from build123d import *

# Parameters (mm, degrees)
F4_R      = 12.7
F5_DEPTH  = 25.4
F7_R      = 12.7
F8_DEPTH  = 25.4
F9_R      = 7.463803
F9_R_2    = 6.828803
F10_DEPTH = 0.635


with BuildPart() as f1:
    # F0 (on Front) → F1 (revolve)
    with BuildSketch(Plane.XZ):
        with BuildLine():
            ThreePointArc((0, -8.048003), (8.048003, 0), (0, 8.048003))
            Line((0, 8.048003), (0, -8.048003))
        make_face()
    revolve(axis=Axis((0, 0, 0), (0, 0, -1)))

    # F2 (on Front) → F3 (revolve, cut)
    with BuildSketch(Plane.XZ):
        with BuildLine():
            ThreePointArc((0, -6.270003), (6.270003, 0), (0, 6.270003))
            Line((0, 6.270003), (0, -6.270003))
        make_face()
    revolve(axis=Axis((0, 0, 0), (0, 0, -1)), mode=Mode.SUBTRACT)

    # F4 (on Top) → F5 (cut)
    with BuildSketch(Plane.XY):
        Circle(F4_R)
    extrude(amount=F5_DEPTH, mode=Mode.SUBTRACT)

    # F7 (on offset) → F8 (cut)
    with BuildSketch(Plane.XY.offset(-3.81)):
        Circle(F7_R)
    extrude(amount=-F8_DEPTH, mode=Mode.SUBTRACT)

    # F9 (on face) → F10 (join)
    with BuildSketch(Plane.XY):
        Circle(F9_R)
        Circle(F9_R_2, mode=Mode.SUBTRACT)
    extrude(amount=F10_DEPTH)


solid = f1.part
Input: part model. Units: mm. Frame: model coordinates. Coordinates: 2 decimals unless noted, no trailing zeros. Loops run counter-clockwise (first coordinate to the right, second up) from the corner with the lowest first, then second, coordinate; pieces in that order, holes last.
Q1. Cut plane A-A (x = 4.75). Output: boundary loops of the cut face in (y, z) (3 decimals).
Q2. Contact query for a flat-ended pin moving along its axis: pin 1 (1 mm diameter, centred on x = 4.5, y = 1, fed in from +Z). Output: stop coordinate, or through.
Q3. Cut plane C-C (z = -2.8). Output: boundary loops of the cut face in (x, y).
Q4. Draft query along Y for faces 1 (the face through (6.308, -2.615, 0.313)), 2 (the face through (5, -6, 0)), 3 (the face through (7.12, 2.24, 0.31)). Return one class per face: +Y half, -Y half, draft (parallel to the pull), parting line (faces both ways), or undercut.
Q5. Material intervals for line 1 (Y direction, x = 0, z = 0.3); line 2 (Y direction, x = -2.5, z = 0.25); line 3 (X direction, y = -5.25, z = -0.85), sorted ascending.
Q6. Cut plane B-B (y = 0.5). Output: boundary loops of the cut face in (x, z) (3 decimals).
Working result:
1. outline: (-6.497, 0) arc R6.497 ccw to (-5.262, -3.81) - (-1.495, -3.81) arc R4.093 cw to (-4.093, 0) - (-4.906, 0) - (-4.906, 0.635) - (-5.757, 0.635) - (-5.757, 0) - close; (1.495, -3.81) - (5.262, -3.81) arc R6.497 ccw to (6.497, 0) - (5.757, 0) - (5.757, 0.635) - (4.906, 0.635) - (4.906, 0) - (4.093, 0) arc R4.093 cw to start
2. pin 1: stops at z = -3.63
3. outline: circle Ø15.09 at (0, 0); hole circle Ø11.22 at (0, 0)
4. face 1: undercut
4. face 2: draft
4. face 3: parting line
5. line 1: y = -7.46 to -6.83, 6.83 to 7.46
5. line 2: y = -7.03 to -6.35, 6.35 to 7.03
5. line 3: x = -6.04 to -3.32, 3.32 to 6.04
6. outline: (-8.032, 0) arc R8.032 ccw to (-7.071, -3.81) - (-4.954, -3.81) arc R6.25 cw to (-6.25, 0) - (-6.81, 0) - (-6.81, 0.635) - (-7.447, 0.635) - (-7.447, 0) - close; (4.954, -3.81) - (7.071, -3.81) arc R8.032 ccw to (8.032, 0) - (7.447, 0) - (7.447, 0.635) - (6.81, 0.635) - (6.81, 0) - (6.25, 0) arc R6.25 cw to start
